Here's how the part is built. I have some questions about the finished solid (model axes, mm). A direction names the side the tool comes from. Give positions to 0.01 mm unless a question says otherwise; leave off trailing zeros. Write each loop counter-clockwise with the first axis right and the second up, starting at its lowest first coordinate (ties: lowest second). Pieces come first, ordered by that corner, then holes. Notation, with made-up numbers: (70, 63.5) -> (95, 63.5) arc R26 cw to (95, 82.5) -> close; hole circle Ø10 at (36, -1.5). An arc over 180 degrees is marked (long way). Return JSON: item names as keys, results as strings.
from build123d import *

# Parameters (mm, degrees)
SKETCH1_W                          = 99.9998
SKETCH1_H                          = 50
MAIN_EXTRUDE_DEPTH                 = 24.003
F_1_8_0_125_DIAMETER_HOLE1_D       = 3.175
F_1_8_0_125_DIAMETER_HOLE1_DEPTH   = 5.08
M3X0_5_TAPPED_HOLE1_D              = 2.5
M3X0_5_TAPPED_HOLE1_DEPTH          = 6.35
CIRPATTERN1_COUNT                  = 3
F_3_16_0_1875_DIAMETER_HOLE1_D     = 4.7625
F_3_16_0_1875_DIAMETER_HOLE1_DEPTH = 6.2484
M3X0_5_TAPPED_HOLE2_D              = 2.5
M3X0_5_TAPPED_HOLE2_DEPTH          = 5.801995
M3X0_5_TAPPED_HOLE2_TIP            = 0.751075774
M5X0_8_TAPPED_HOLE2_D              = 4.2
M5X0_8_TAPPED_HOLE2_DEPTH          = 12.7
M5X0_8_TAPPED_HOLE2_TIP            = 1.2618073
M5X0_8_TAPPED_HOLE1_D              = 4.2
CHAMFER1_SIZE                      = 0.762
EXTRUDE1_DEPTH                     = 0.9398
EXTRUDE2_DEPTH                     = 2.49936


with BuildPart() as part:
    # Sketch1 → Main Extrude (new body)
    with BuildSketch(Plane(origin=(0, 0, 0), x_dir=(1, 0, 0), z_dir=(0, 1, 0))):
        Rectangle(SKETCH1_W, SKETCH1_H)
    extrude(amount=MAIN_EXTRUDE_DEPTH)

    # 1_8 _0.125_ Diameter Hole1
    with Locations(Plane.XZ):
        with Locations((-24.9999, 0)):
            Hole(F_1_8_0_125_DIAMETER_HOLE1_D / 2, depth=F_1_8_0_125_DIAMETER_HOLE1_DEPTH)

    # M3x0.5 Tapped Hole1
    with Locations(Plane.XZ):
        with Locations((10.795, 0)):
            m3x0_5_tapped_hole1 = Hole(M3X0_5_TAPPED_HOLE1_D / 2, depth=M3X0_5_TAPPED_HOLE1_DEPTH)

    # CirPattern1: M3x0.5 Tapped Hole1 ×3 about axis
    cirpattern1_axis = Axis((0, 0, 0), (0, 1, 0))
    for i in range(1, CIRPATTERN1_COUNT):
        add(m3x0_5_tapped_hole1.rotate(cirpattern1_axis, i * 360 / CIRPATTERN1_COUNT), mode=Mode.SUBTRACT)

    # 3_16 _0.1875_ Diameter Hole1
    with Locations(Plane.XZ):
        with Locations((0, 0)):
            Hole(F_3_16_0_1875_DIAMETER_HOLE1_D / 2, depth=F_3_16_0_1875_DIAMETER_HOLE1_DEPTH)

    # Sketch12 → Cut-Revolve1 (revolve, cut)
    with BuildSketch(Plane.XZ.offset(0.508)):
        with BuildLine():
            Line((0, 6.5024), (0, -6.5024))
            ThreePointArc((0, -6.5024), (6.5024, 0), (0, 6.5024))
        make_face()
    revolve(axis=Axis((0, -0.508, 6.5024), (0, 0, -1)), mode=Mode.SUBTRACT)

    # M3x0.5 Tapped Hole2
    with Locations(Plane.XZ):
        with Locations((25.0001, 0)):
            Hole(M3X0_5_TAPPED_HOLE2_D / 2, depth=M3X0_5_TAPPED_HOLE2_DEPTH)
            with Locations((0, 0, -(M3X0_5_TAPPED_HOLE2_DEPTH + M3X0_5_TAPPED_HOLE2_TIP / 2))):  # 118° drill point
                Cone(0, M3X0_5_TAPPED_HOLE2_D / 2, M3X0_5_TAPPED_HOLE2_TIP, mode=Mode.SUBTRACT)

    # M5x0.8 Tapped Hole2
    with Locations(Plane(origin=(49.9999, 0, 0), x_dir=(0, 0, -1), z_dir=(1, 0, 0))):
        with Locations((0, 15.748)):
            Hole(M5X0_8_TAPPED_HOLE2_D / 2, depth=M5X0_8_TAPPED_HOLE2_DEPTH)
            with Locations((0, 0, -(M5X0_8_TAPPED_HOLE2_DEPTH + M5X0_8_TAPPED_HOLE2_TIP / 2))):  # 118° drill point
                Cone(0, M5X0_8_TAPPED_HOLE2_D / 2, M5X0_8_TAPPED_HOLE2_TIP, mode=Mode.SUBTRACT)

    # M5x0.8 Tapped Hole1 (through all)
    with Locations(Plane.XZ):
        with Locations((41.3131, 0)):
            Hole(M5X0_8_TAPPED_HOLE1_D / 2)

    # Chamfer1
    chamfer1_edges = [part.edges().sort_by_distance(p)[0] for p in [
        (0, 0, -25),
        (49.9999, 0, 0),
        (0, 0, 25),
        (-49.9999, 0, 0),
    ]]
    chamfer(chamfer1_edges, length=CHAMFER1_SIZE)

    # Sketch2 → Extrude1 (add)
    with BuildSketch(Plane(origin=(0, 24.003, 0), x_dir=(-1, 0, 0), z_dir=(0, 1, 0))):
        with BuildLine():
            Line((45.8724, 24.0475), (-45.8724, 24.0475))
            ThreePointArc((-45.8724, 24.0475), (-48.11746403, 23.11756403), (-49.0474, 20.8725))
            Line((-49.0474, 20.8725), (-49.0474, -20.8851))
            ThreePointArc((-49.0474, -20.8851), (-48.11746403, -23.13016403), (-45.8724, -24.0601))
            Line((-45.8724, -24.0601), (45.8724, -24.0601))
            ThreePointArc((45.8724, -24.0601), (48.11746403, -23.13016403), (49.0474, -20.8851))
            Line((49.0474, -20.8851), (49.0474, 20.8725))
            ThreePointArc((49.0474, 20.8725), (48.11746403, 23.11756403), (45.8724, 24.0475))
        make_face()
    extrude(amount=EXTRUDE1_DEPTH)

    # Sketch19 → Extrude2 (add)
    with BuildSketch(Plane.XZ):
        Polygon((36.693720496, 0), (39.003410248, -4.0005), (43.622789752, -4.0005), (45.932479504, 0), (43.622789752, 4.0005), (39.003410248, 4.0005), align=None)
    extrude(amount=EXTRUDE2_DEPTH)


solid = part.part
1. Suppose I cut it at B-B, the plane z = 15. List the corners of the cut face in (x, y) for me, and give its area (3 significant figures).
Taken from the geometry:
{"outline": "(-50, 0.76) -> (-49.24, 0) -> (49.24, 0) -> (50, 0.76) -> (50, 24) -> (49.05, 24) -> (49.05, 24.94) -> (-49.05, 24.94) -> (-49.05, 24) -> (-50, 24) -> close", "area": "2,490 mm²"}
2. Suppose I cut it at A-A, the plane x = 0. List the corners of the cut face in (y, z) for me, and give its area (3 significant figures).
Taken from the geometry:
{"outline": "(0, -24.24) -> (0.76, -25) -> (24, -25) -> (24, -24.06) -> (24.94, -24.06) -> (24.94, 24.05) -> (24, 24.05) -> (24, 25) -> (0.76, 25) -> (0, 24.24) -> (0, 6.48) arc R6.5 cw to (5.54, 2.38) -> (6.25, 2.38) -> (6.25, -2.38) -> (5.54, -2.38) arc R6.5 cw to (0, -6.48) -> close", "area": "1,180 mm²"}
3. If we mould it in two halves opening along Z, with no side actions, what happens to faces 1 (the face through (-48.093, 24.466, -23.155)), 2 (the face through (11, 6.35, 0)), 3 (the face through (23.845, 2.942, -0.479)), 4 (the face through (-48.142, 24.466, 23.093))? For each: released by +Z, released by -Z, zero draft, split by the parting line, or undercut.
Taken from the geometry:
{"face 1": "released by -Z", "face 2": "undercut", "face 3": "undercut", "face 4": "released by +Z"}
4. For pin 1 Ø8 at (x, z) = (16, 12.5) entering from -Y; pin 2 Ø0.8 at (y, z) = (24.5, -2.5) entering from -X; pin 3 Ø2.5 at (x, y) = (41, -1) entering from +Z, each with a flat end and sliding along its axis, tell me the tip position at first contact or that it passes through.
Taken from the geometry:
{"pin 1": "stops at y = 0", "pin 2": "stops at x = -49.05", "pin 3": "stops at z = 24.49"}
5. If I drill on line 1 (Z direction, x = 0, y = 5.85); line 2 (Y direction, x = 40, z = 0); line 3 (Y direction, x = 33.5, z = -0.5), over which ranges is the centre line in solid material (lowest first)? Write a range as [from, to].
Taken from the geometry:
{"line 1": "z = [-25, -2.38], [2.38, 25]", "line 2": "y = [-2.5, 0], [24, 24.94]", "line 3": "y = [0, 24.94]"}
6. Suppose I cut it at C-C, the plane x = -12.5. List the corners of the cut face in (y, z) for me.
Taken from the geometry:
{"outline": "(0, -24.24) -> (0.76, -25) -> (24, -25) -> (24, -24.06) -> (24.94, -24.06) -> (24.94, 24.05) -> (24, 24.05) -> (24, 25) -> (0.76, 25) -> (0, 24.24) -> close"}
7. Which directions (+Z, -Z, +X, -X, +Y, -Y) give clear straight access to the entire face, cutting with the end or side of a thin tool? Please do faces 5 (the face through (41, 0, 0)), 6 (the face through (44.794, -1.232, 1.972)), 7 (the face through (-25, 5.08, 0)), 8 (the face through (38.832, 17.167, -1.548)).
Taken from the geometry:
{"face 5": "none", "face 6": "+Z, +X, -Y", "face 7": "-Y", "face 8": "+X"}
